```python
from build123d import *

# Parameters (mm, degrees)
F0_W     = 152.4
F0_H     = 63.5
F1_DEPTH = 3.175
F2_W     = 142.875
F2_H     = 53.975
F3_DEPTH = 3.175
F4_R     = 4.7625
F5_T     = -3.175


with BuildPart() as f1:
    # F0 (on Top) → F1 (new body)
    with BuildSketch(Plane.XY):
        Rectangle(F0_W, F0_H)
    extrude(amount=F1_DEPTH)

    # F2 (on face) → F3 (join)
    with BuildSketch(Plane.XY.offset(3.175)):
        Rectangle(F2_W, F2_H)
    extrude(amount=F3_DEPTH)

    # F4
    f4_edges = [f1.edges().sort_by_distance(p)[0] for p in [
        (71.4375, -26.9875, 4.7625),
        (71.4375, 26.9875, 4.7625),
        (-71.4375, -26.9875, 4.7625),
        (76.2, -31.75, 1.5875),
        (76.2, 31.75, 1.5875),
        (-76.2, -31.75, 1.5875),
        (-71.4375, 26.9875, 4.7625),
        (-76.2, 31.75, 1.5875),
    ]]
    fillet(f4_edges, radius=F4_R)

    # F5
    f5_openings = [f1.faces().sort_by_distance(p)[0] for p in [
        (0, 0, 6.35),
    ]]
    offset(amount=F5_T, openings=f5_openings, kind=Kind.INTERSECTION)


solid = f1.part
```
Geometry: final body of the model. Coordinates: model frame, mm. A direction names the side the tool comes from. Round coordinates to 2 decimals unless told otherwise and drop trailing zeros. Loops run counter-clockwise (first coordinate to the right, second up) from the corner with the lowest first, then second, coordinate; pieces in that order, holes last.
Item 1: Section A-A, the plane z = 5. Output: boundary loops of the cut face in (x, y) (1 decimal).
Checked values:
outline: (-71.4, -22.2) arc R4.8 ccw to (-66.7, -27) - (66.7, -27) arc R4.8 ccw to (71.4, -22.2) - (71.4, 22.2) arc R4.8 ccw to (66.7, 27) - (-66.7, 27) arc R4.8 ccw to (-71.4, 22.2) - close; hole (-68.3, -22.2) arc R1.6 ccw to (-66.7, -23.8) - (66.7, -23.8) arc R1.6 ccw to (68.3, -22.2) - (68.3, 22.2) arc R1.6 ccw to (66.7, 23.8) - (-66.7, 23.8) arc R1.6 ccw to (-68.3, 22.2) - close
Item 2: Contact query for flat-ended pins moving along their axis: P1, Ø1.6, axis at y = -2.5, z = 4.5, coming from the +X side; P2, Ø2.5, axis at x = 5.5, z = 4.5, coming from the -Y side; P3, Ø1, axis at x = 40, y = 1, coming from the +Z side (3 decimals). Output: stop coordinate, or through.
Checked values:
P1: stops at x = 71.44
P2: stops at y = -26.99
P3: stops at z = 3.175
Item 3: Reachability of faces 1 (the flat face through (71.438, 0, 5)), 2 (the cylindrical face through (-70.005, -25.629, 4.785)), 3 (the cylindrical face through (70.079, 25.555, 4.785)), 4 (the flat face through (-1, -26.988, 5)), 5 (the flat face through (-6, -28, 3.175)) from +Z, -Z, +X, -X, +Y, -Y: full face, straight path, thin tool, end or side. Return the list, or none.
Checked values:
face 1: +Z, +X, +Y, -Y
face 2: +Z, -X, -Y
face 3: +Z, +X, +Y
face 4: +Z, +X, -X, -Y
face 5: +Z
Item 4: Mould query, pull axis X, two halves, no side actions, for faces 6 (the flat face through (-1, 23.812, 5)), 7 (the flat face through (-76.2, 0, 2)), 8 (the flat face through (-1, 31.75, 2)). Classes: released by +X, released by -X, zero draft, split by the parting line, or undercut.
Checked values:
face 6: undercut
face 7: released by -X
face 8: zero draft
Item 5: Line query: L1, parallel to X at y = 18.5, z = 4.25; L2, parallel to Y at x = -28.5, z = 5; L3, parallel to Z at x = 8, y = 9 (3 decimals). Output: solid intervals per line, ascending.
Checked values:
L1: x = -71.44 to -68.26, 68.26 to 71.44
L2: y = -26.99 to -23.81, 23.81 to 26.99
L3: z = 0 to 3.175
